Source: CAD feature listing. Evaluate the final solid. Frame: model axes, mm. Face numbers are marked on the shaded views. Coordinates: 2 decimals unless noted, no trailing zeros. Write each loop counter-clockwise with the first axis right and the second up, starting at its lowest first coordinate (ties: lowest second). Pieces come first, ordered by that corner, then holes. Notation, with made-up numbers: M 43,36 L 77,36 A23 ccw 77,54 Z; hole C 71.25,70.5 d5. An arc over 180 degrees is marked long. Write item = value, one per line. Start each with the question number.
1. Pull-direction query (X, two-part tool) for the marked faces 1 and 2; classes: pulls with the +X half, pulls with the -X half, needs draft (parallel to the pull), parting line crosses it, or undercut.
2. Line query: line 1 along X through (y, z) = (4, 2.5); line 2 along Z through (x, y) = (-2, 5); line 3 along Z through (x, y) = (-23, 4.25). Output: solid intervals per line, ascending.
3. Section query B-B (z = 4.5). Output: boundary loops of the cut face in (x, y).
4. Section query C-C (z = -14.5). Output: boundary loops of the cut face in (x, y), then the cut area to 3 significant figures.
5. Section query D-D (y = 0.75). Give the number of separate pieces and of enclosed holes in the cut face, then the cut area to 3 significant figures.
6. Section query A-A (x = 0). Output: boundary loops of the cut face in (y, z).
7. Pin query (flat end, axial travel): pin 1 Ø3 at (y, z) = (0.5, 14) entering from -X; pin 2 Ø1 at (x, z) = (0.5, 20.5) entering from -Y; pin 3 Ø3 at (x, y) = (-10, 1.5) entering from -Z. Return the tip coordinate at first contact, or that it passes through.
```python
from build123d import *

# Parameters (mm, degrees)
SKETCH1_R                   = 31.6865
BOSS_EXTRUDE1_DEPTH         = 6.35
CIRPATTERN1_COUNT           = 4
SKETCH5_W                   = 1.2954
SKETCH5_H                   = 2.413
F_3_4_CLEARANCE_HOLE1_D     = 19.44624
F_3_4_CLEARANCE_HOLE1_DEPTH = 6.35
F_3_4_CLEARANCE_HOLE1_TIP   = 5.842239902


with BuildPart() as part:
    # Sketch1 → Boss-Extrude1 (new body)
    with BuildSketch(Plane(origin=(0, 0, 0), x_dir=(1, 0, 0), z_dir=(0, 1, 0))):
        with Locations(Location((0, 0, 0), (0, 0, 270))):
            Circle(SKETCH1_R)
    extrude(amount=BOSS_EXTRUDE1_DEPTH)

    # Sketch4 → Cut-Revolve1 (revolve, cut)
    with BuildSketch(Plane.XY, mode=Mode.PRIVATE) as cut_revolve1_sk:
        Polygon((-28.472660076, 8.787660076), (-22.86, 3.175), (-17.247339924, -2.437660076), (-15.092078455, -0.282398607), (-26.317398607, 10.942921545), align=None)
    cut_revolve1 = revolve(cut_revolve1_sk.sketch.rotate(Axis((-28.472660076, 8.787660076, 0), (0.7071067811865512, -0.7071067811865439, 0)), 180), axis=Axis((-28.472660076, 8.787660076, 0), (0.7071067811865512, -0.7071067811865439, 0)), mode=Mode.SUBTRACT)

    # CirPattern1: Cut-Revolve1 ×4 about axis
    cirpattern1_axis = Axis((0, -0.3175, 0), (0, 1, 0))
    for i in range(1, CIRPATTERN1_COUNT):
        add(cut_revolve1.rotate(cirpattern1_axis, i * 360 / CIRPATTERN1_COUNT), mode=Mode.SUBTRACT)

    # Sketch5 → Cut-Revolve2 (revolve, cut)
    with BuildSketch(Plane.XY, mode=Mode.PRIVATE) as cut_revolve2_sk:
        with Locations((31.0388, 3.3655)):
            Rectangle(SKETCH5_W, SKETCH5_H)
    revolve(cut_revolve2_sk.sketch.rotate(Axis((0, -0.3175, 0), (0, 1, 0)), 90), axis=Axis((0, -0.3175, 0), (0, 1, 0)), mode=Mode.SUBTRACT)

    # 3/4 Clearance Hole1
    with Locations(Plane(origin=(0, 6.35, 0), x_dir=(1, 0, 0), z_dir=(0, 1, 0))):
        with Locations((0, 0)):
            Hole(F_3_4_CLEARANCE_HOLE1_D / 2, depth=F_3_4_CLEARANCE_HOLE1_DEPTH)
            with Locations((0, 0, -(F_3_4_CLEARANCE_HOLE1_DEPTH + F_3_4_CLEARANCE_HOLE1_TIP / 2))):  # 118° drill point
                Cone(0, F_3_4_CLEARANCE_HOLE1_D / 2, F_3_4_CLEARANCE_HOLE1_TIP, mode=Mode.SUBTRACT)


solid = part.part
```
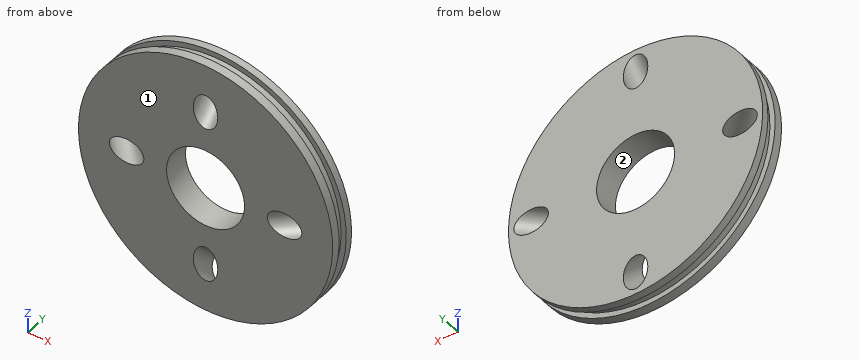
Results are:
q1.face_1 = needs draft
q1.face_2 = undercut
q2.line_1 = -30.29 to -26.15, -21.22 to -9.4, 9.4 to 21.22, 26.15 to 30.29
q2.line_2 = -31.62 to -27.94, -21.43 to -9.52, 9.52 to 21.43, 27.94 to 31.62
q2.line_3 = -19.87 to -2.98, 2.98 to 19.87
q3.outline = M -31.37,0 L -8.62,0 L -8.62,6.35 L -31.37,6.35 L -31.37,4.57 L -30.06,4.57 L -30.06,2.16 L -31.37,2.16 Z; M 8.62,0 L 31.37,0 L 31.37,2.16 L 30.06,2.16 L 30.06,4.57 L 31.37,4.57 L 31.37,6.35 L 8.62,6.35 Z
q4.outline = M -28.17,0 L 28.17,0 L 28.17,2.16 L 26.71,2.16 L 26.71,4.57 L 28.17,4.57 L 28.17,6.35 L -28.17,6.35 L -28.17,4.57 L -26.71,4.57 L -26.71,2.16 L -28.17,2.16 Z
q4.area = 351 mm^2
q5.separate_pieces = 1
q5.enclosed_holes = 5
q5.area = 2,690 mm^2
q6.outline = M 0,-31.69 L 2.16,-31.69 L 2.16,-30.39 L 4.57,-30.39 L 4.57,-31.69 L 6.35,-31.69 L 6.35,-30.35 L 0,-24 Z; M 0,-15.37 L 6.35,-21.72 L 6.35,-9.72 L 0,-9.72 Z; M 0,9.72 L 6.35,9.72 L 6.35,21.72 L 0,15.37 Z; M 0,24 L 6.35,30.35 L 6.35,31.69 L 4.57,31.69 L 4.57,30.39 L 2.16,30.39 L 2.16,31.69 L 0,31.69 Z
q7.pin_1 = -29.12
q7.pin_2 = 4.55
q7.pin_3 = -30.53
